```python
from build123d import *

# Parameters (mm, degrees)
SKETCH1_R           = 2.5
BOSS_EXTRUDE2_DEPTH = 1


with BuildPart() as part:
    # Sketch1 → Boss-Extrude2 (new body)
    with BuildSketch(Plane.XY):
        Polygon((3, 173), (0, 173), (0, 43), (3, 43), (3, 33), (0, 33), (0, 23), (3, 23), (3, 13), (0, 13), (0, 3), (10, 3), (10, 0), (20, 0), (20, 3), (40, 3), (40, 0), (50, 0), (50, 3), (57, 3), (57, 23), (60, 23), (60, 33), (57, 33), (57, 53), (60, 53), (60, 63), (57, 63), (57, 83), (60, 83), (60, 93), (57, 93), (57, 123), (60, 123), (60, 133), (57, 133), (57, 153), (60, 153), (60, 163), (57, 163), (57, 183), (60, 183), (60, 193), (57, 193), (57, 213), (50, 213), (50, 216), (40, 216), (40, 213), (20, 213), (20, 216), (10, 216), (10, 213), (0, 213), (0, 203), (3, 203), (3, 193), (0, 193), (0, 183), (3, 183), align=None)
        with Locations((12, 15)):
            Circle(SKETCH1_R, mode=Mode.SUBTRACT)
        with Locations((10, 30)):
            Circle(SKETCH1_R, mode=Mode.SUBTRACT)
        with BuildLine():
            ThreePointArc((24, 18), (24.878679656, 20.121320344), (27, 21))
            Line((27, 21), (51, 21))
            ThreePointArc((51, 21), (53.121320344, 20.121320344), (54, 18))
            Line((54, 18), (54, 9))
            ThreePointArc((54, 9), (53.121320344, 6.878679656), (51, 6))
            Line((51, 6), (27, 6))
            ThreePointArc((27, 6), (24.878679656, 6.878679656), (24, 9))
            Line((24, 9), (24, 18))
        make_face(mode=Mode.SUBTRACT)
        with Locations((8, 205)):
            Circle(SKETCH1_R, mode=Mode.SUBTRACT)
        with Locations((37, 151)):
            Circle(SKETCH1_R, mode=Mode.SUBTRACT)
        with Locations((34.713021846, 189.185576425)):
            Circle(SKETCH1_R, mode=Mode.SUBTRACT)
    extrude(amount=BOSS_EXTRUDE2_DEPTH)


solid = part.part
```
For this review, take the finished solid that the model builds, in its own axes (mm). Round coordinates to 2 decimals unless told otherwise and drop trailing zeros. Write each loop counter-clockwise with the first axis right and the second up, starting at its lowest first coordinate (ties: lowest second). Pieces come first, ordered by that corner, then holes. Notation, with made-up numbers: (10, 38) - (28, 38) arc R29 cw to (28, 69) - close; hole circle Ø11 at (48.5, 23). An arc over 180 degrees is marked (long way). Answer as CSV lines item,"result". Start each with the question number.
(1) Add section A-A, the plane y = 30. State the section outline as (x, z) points, plus the area to 3 significant figures.
(2) Add section D-D, the plane y = 197. State the section outline as (x, z) points, plus the area to 3 significant figures.
(3) Add section B-B, the plane y = 151. State the section outline as (x, z) points.
(4) For line 1 (X direction, y = 205, z = 0.3); line 2 (Y direction, x = 8, z = 0.4); line 3 (Y direction, x = 42, z = 0.9), list the stretches that pass through material, from the lowest coordinate up.
(5) For pin 1 (0.5 mm diameter, centred on x = 54, z = 0.5, fed in from -Y); pin 2 (0.5 mm diameter, centred on y = 178.5, z = 0.5, fed in from -X); pin 3 (0.5 mm diameter, centred on y = 2, z = 0.5, fed in from +X), all flat-tipped, find the tip position at first contact; note any pin that passes through.
(6) Mouldability with a two-part tool opening along Y and no side actions: class faces 1 (the flat face through (30, 110, 1)), 2 (the cylindrical face through (7.67, 207.48, 0.49)), 3 (the cylindrical face through (11.34, 32.11, 0.49)) as +Y half, -Y half, draft (parallel to the pull), parting line (faces both ways), or undercut.
(7) Add section C-C, the plane z = 0.8. State how many separate pieces and enclosed holes the cut face has, plus the area to 3 significant figures.
From the geometry:
1,outline,"(0, 0) - (7.5, 0) - (7.5, 1) - (0, 1) - close; (12.5, 0) - (60, 0) - (60, 1) - (12.5, 1) - close"
1,area,"55.0 mm²"
2,outline,"(3, 0) - (57, 0) - (57, 1) - (3, 1) - close"
2,area,"54.0 mm²"
3,outline,"(0, 0) - (34.5, 0) - (34.5, 1) - (0, 1) - close; (39.5, 0) - (57, 0) - (57, 1) - (39.5, 1) - close"
4,line 1,"x = 0 to 5.5, 10.5 to 57"
4,line 2,"y = 3 to 28.5, 31.5 to 202.5, 207.5 to 213"
4,line 3,"y = 0 to 6, 21 to 216"
5,pin 1,"stops at y = 3"
5,pin 2,"stops at x = 3"
5,pin 3,"stops at x = 50"
6,face 1,"draft"
6,face 2,"undercut"
6,face 3,"undercut"
7,separate pieces,"1"
7,enclosed holes,"6"
7,area,"11,600 mm²"
